The listing builds one solid part. Answer for the finished solid, in the listing's coordinates (mm). Face numbers are marked on the shaded views. A direction names the side the tool comes from. Coordinates: 2 decimals unless noted, no trailing zeros. Loops run counter-clockwise (first coordinate to the right, second up) from the corner with the lowest first, then second, coordinate; pieces in that order, holes last. Notation, with made-up numbers: M -32,17.25 L 8,17.25 A24 ccw 8,29.25 Z; hole C -30.5,15 d10. An arc over 180 degrees is marked long. Answer as CSV lines item,"result". Start each with the question number.
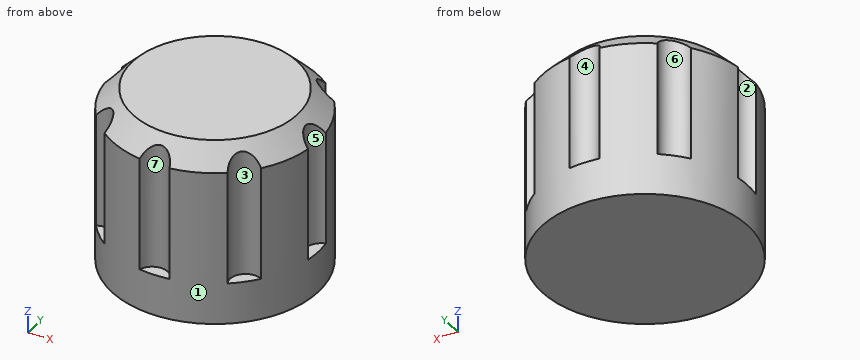
```python
from build123d import *

# Parameters (mm, degrees)
CYLINDER001_R     = 1.5
CYLINDER001_DEPTH = 15
ARRAY_COUNT       = 8
CYLINDER_R        = 10
CYLINDER_DEPTH    = 17
CHAMFER_SIZE      = 2


with BuildPart() as array:
    # Cylinder001 → Cylinder001 (new body)
    with BuildSketch(Plane(origin=(0.2, 0, 12), x_dir=(1, 0, 0), z_dir=(0, 0, 1))):
        Circle(CYLINDER001_R)
    extrude(amount=CYLINDER001_DEPTH)

    # Array: Array ×8 about axis
    array_axis = Axis((10.5, 0, 0), (0, 0, 1))


with BuildPart() as array_1:
    add(array.part)
    for i in range(1, ARRAY_COUNT):
        add(array.part.rotate(array_axis, i * 360 / ARRAY_COUNT))


with BuildPart() as cut:
    # Cylinder → Cylinder (new body)
    with BuildSketch(Plane(origin=(10.5, 0, 8), x_dir=(1, 0, 0), z_dir=(0, 0, 1))):
        Circle(CYLINDER_R)
    extrude(amount=CYLINDER_DEPTH)

    # Chamfer
    chamfer_edges = [cut.edges().sort_by_distance(p)[0] for p in [
        (0.5, 0, 25),
    ]]
    chamfer(chamfer_edges, length=CHAMFER_SIZE)

    # Cut: cut Array
    add(array_1.part, mode=Mode.SUBTRACT)


solid = cut.part
```
Item 1: For the marked faces 4, 5, 6 and 7, determine the directions among +Z, -Z, +X, -X, +Y, -Y from which every point of the face is accessible in a straight line to the end or side of a thin tool.
Item 2: Section A-A on x = 10.5 is taken. Determine the outline of the cut face in (y, z), then the cut area to 3 significant figures.
Item 3: Section C-C on z = 19.5 is taken. Determine the outline of the cut face in (x, y).
Item 4: Each of these flat-tipped pins is pushed along its axis until it touches: P1, Ø0.6, axis at x = 1.5, y = 0.5, coming from the +Z side; P2, Ø4, axis at x = 16.5, z = 10.5, coming from the -Y side; P3, Ø0.7, axis at x = 3, y = -7.5, coming from the +Z side; P4, Ø1, axis at x = 20, y = 0, coming from the +Z side. Where does it stop, or does it pass through?
Item 5: For a pull along X with two mould halves and no side action, classify the marked faces 1, 2 and 3 as pulls with the +X half, pulls with the -X half, needs draft (parallel to the pull), parting line crosses it, or undercut.
Item 6: Consider line 1 (Y direction, x = 17.75, z = 15.5); line 2 (X direction, y = -6, z = 9.25); line 3 (Z direction, x = 4, y = -6.25). Determine where each line is inside the solid, lowest interval first.
Item 7: Section B-B on y = 0 is taken. Determine the outline of the cut face in (x, z).
Results are:
1,face 4,"+Z, +Y"
1,face 5,"+Z, +X"
1,face 6,"+Z"
1,face 7,"+Z, -Y"
2,outline,"M -10,8 L 10,8 L 10,12 L 8.8,12 L 8.8,24.2 L 8,25 L -8,25 L -8.8,24.2 L -8.8,12 L -10,12 Z"
2,area,"308 mm²"
3,outline,"M 0.6,-1.44 A10 ccw 2.48,-5.98 A1.5 cw 4.52,-8.02 A10 ccw 9.06,-9.9 A1.5 cw 11.94,-9.9 A10 ccw 16.48,-8.02 A1.5 cw 18.52,-5.98 A10 ccw 20.4,-1.44 A1.5 cw 20.4,1.44 A10 ccw 18.52,5.98 A1.5 cw 16.48,8.02 A10 ccw 11.94,9.9 A1.5 cw 9.06,9.9 A10 ccw 4.52,8.02 A1.5 cw 2.48,5.98 A10 ccw 0.6,1.44 A1.5 cw Z"
4,P1,"z = 24.29"
4,P2,"y = -9.17"
4,P3,"through"
4,P4,"z = 12"
5,face 1,"parting line crosses it"
5,face 2,"pulls with the -X half"
5,face 3,"undercut"
6,line 1,"-5.78 to 5.78"
6,line 2,"2.5 to 18.5"
6,line 3,"8 to 12"
7,outline,"M 0.5,8 L 20.5,8 L 20.5,12 L 19.3,12 L 19.3,24.2 L 18.5,25 L 2.5,25 L 1.7,24.2 L 1.7,12 L 0.5,12 Z"
